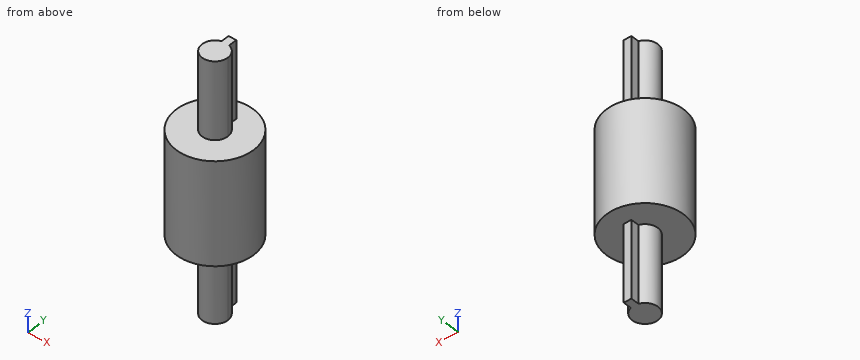
from build123d import *

# Parameters (mm, degrees)
EXTRUDE_1_DEPTH = 30
SKETCH_2_R      = 15
EXTRUDE_2_DEPTH = 25
EXTRUDE_3_DEPTH = 30
SKETCH_4_R      = 15
EXTRUDE_4_DEPTH = 15
EXTRUDE_5_DEPTH = 15


with BuildPart() as part:
    # 草图1 → 凸台-拉伸1 (new body)
    with BuildSketch(Plane.XY):
        with BuildLine():
            Line((-1.5, 8), (-1.5, 4.769696007))
            ThreePointArc((-1.5, 4.769696007), (0, 5), (1.5, 4.769696007))
            Line((1.5, 4.769696007), (1.5, 8))
            Line((1.5, 8), (-1.5, 8))
        make_face()
        with BuildLine():
            Line((1.5, 0), (0, 0))
            Line((0, 0), (-1.5, 0))
            Line((-1.5, 0), (-1.5, 4.769696007))
            ThreePointArc((-1.5, 4.769696007), (-2.958039892, -4.031128874), (5, 0))
            ThreePointArc((5, 0), (4.031128874, 2.958039892), (1.5, 4.769696007))
            Line((1.5, 4.769696007), (1.5, 0))
        make_face()
        with BuildLine():
            Line((-1.5, 0), (0, 0))
            Line((0, 0), (1.5, 0))
            Line((1.5, 0), (1.5, 4.769696007))
            ThreePointArc((1.5, 4.769696007), (0, 5), (-1.5, 4.769696007))
            Line((-1.5, 4.769696007), (-1.5, 0))
        make_face()
    extrude(amount=EXTRUDE_1_DEPTH)

    # 草图2 → 凸台-拉伸2 (add)
    with BuildSketch(Plane.XY.offset(30)):
        Circle(SKETCH_2_R)
    extrude(amount=EXTRUDE_2_DEPTH)

    # 草图3 → 凸台-拉伸3 (add)
    with BuildSketch(Plane.XY.offset(55)):
        with BuildLine():
            Line((1.5, 0), (0, 0))
            Line((0, 0), (-1.5, 0))
            Line((-1.5, 0), (-1.5, 4.769696007))
            ThreePointArc((-1.5, 4.769696007), (-2.958039892, -4.031128874), (5, 0))
            ThreePointArc((5, 0), (4.031128874, 2.958039892), (1.5, 4.769696007))
            Line((1.5, 4.769696007), (1.5, 0))
        make_face()
        with BuildLine():
            Line((-1.5, 0), (0, 0))
            Line((0, 0), (1.5, 0))
            Line((1.5, 0), (1.5, 4.769696007))
            ThreePointArc((1.5, 4.769696007), (0, 5), (-1.5, 4.769696007))
            Line((-1.5, 4.769696007), (-1.5, 0))
        make_face()
        with BuildLine():
            Line((-1.5, 8), (-1.5, 4.769696007))
            ThreePointArc((-1.5, 4.769696007), (0, 5), (1.5, 4.769696007))
            Line((1.5, 4.769696007), (1.5, 8))
            Line((1.5, 8), (-1.5, 8))
        make_face()
    extrude(amount=EXTRUDE_3_DEPTH)

    # 草图4 → 凸台-拉伸4 (add)
    with BuildSketch(Plane.XY.offset(55)):
        Circle(SKETCH_4_R)
    extrude(amount=EXTRUDE_4_DEPTH)

    # 草图5 → 凸台-拉伸5 (add)
    with BuildSketch(Plane.XY.offset(85)):
        with BuildLine():
            ThreePointArc((1.5, 4.769696007), (0, 5), (-1.5, 4.769696007))
            ThreePointArc((-1.5, 4.769696007), (-2.958039892, -4.031128874), (5, 0))
            ThreePointArc((5, 0), (4.031128874, 2.958039892), (1.5, 4.769696007))
        make_face()
        with BuildLine():
            Line((1.5, 8), (-1.5, 8))
            Line((-1.5, 8), (-1.5, 4.769696007))
            ThreePointArc((-1.5, 4.769696007), (0, 5), (1.5, 4.769696007))
            Line((1.5, 4.769696007), (1.5, 8))
        make_face()
    extrude(amount=EXTRUDE_5_DEPTH)


solid = part.part
Geometry check sheet. Reference: the model listing, model coordinates, mm. Give positions to 0.01 mm unless a question says otherwise; leave off trailing zeros. Write each loop counter-clockwise with the first axis right and the second up, starting at its lowest first coordinate (ties: lowest second). Pieces come first, ordered by that corner, then holes. Notation, with made-up numbers: M 7,24 L 43,24 A13 ccw 43,39 Z; hole C 15,60 d4. An arc over 180 degrees is marked long. One line per question, with ' | ' between items.
1. Scan lines: line 1 along Z through (x, y) = (-13, 2.75); line 2 along X through (y, z) = (5.25, 86.5); line 3 along Y through (x, z) = (0, 64.5). Record each from-to range of solid material in increasing order. Write a range as from..to.
Ans:
line 1: 30..70 | line 2: -1.5..1.5 | line 3: -15..15
2. Gauge pin test, flat ends, axial feed: pin 1 (8 mm diameter, centred on y = 10.5, z = 20.5, fed in from -X); pin 2 (10 mm diameter, centred on y = -10.5, z = 53, fed in from +X); pin 3 (10 mm diameter, centred on x = -1, y = 11, fed in from +Z); pin 4 (2.5 mm diameter, centred on y = 5.5, z = 8, fed in from +X). Record the tip position at first contact, or that the pin passes through.
Ans:
pin 1: x = -1.5 | pin 2: x = 13.96 | pin 3: z = 100 | pin 4: x = 2.63
3. Cross-section at C-C (x = 6.75). Enter the section's corners in (y, z), plus the area to 3 significant figures.
Ans:
outline: M -13.4,30 L 13.4,30 L 13.4,70 L -13.4,70 Z | area: 1,070 mm2
4. Cross-section at A-A (z = 57). Enter the section's corners in (x, y).
Ans:
outline: C 0,0 d30
5. Cross-section at B-B (y = -12). Enter the section's corners in (x, z).
Ans:
outline: M -9,30 L 9,30 L 9,70 L -9,70 Z
